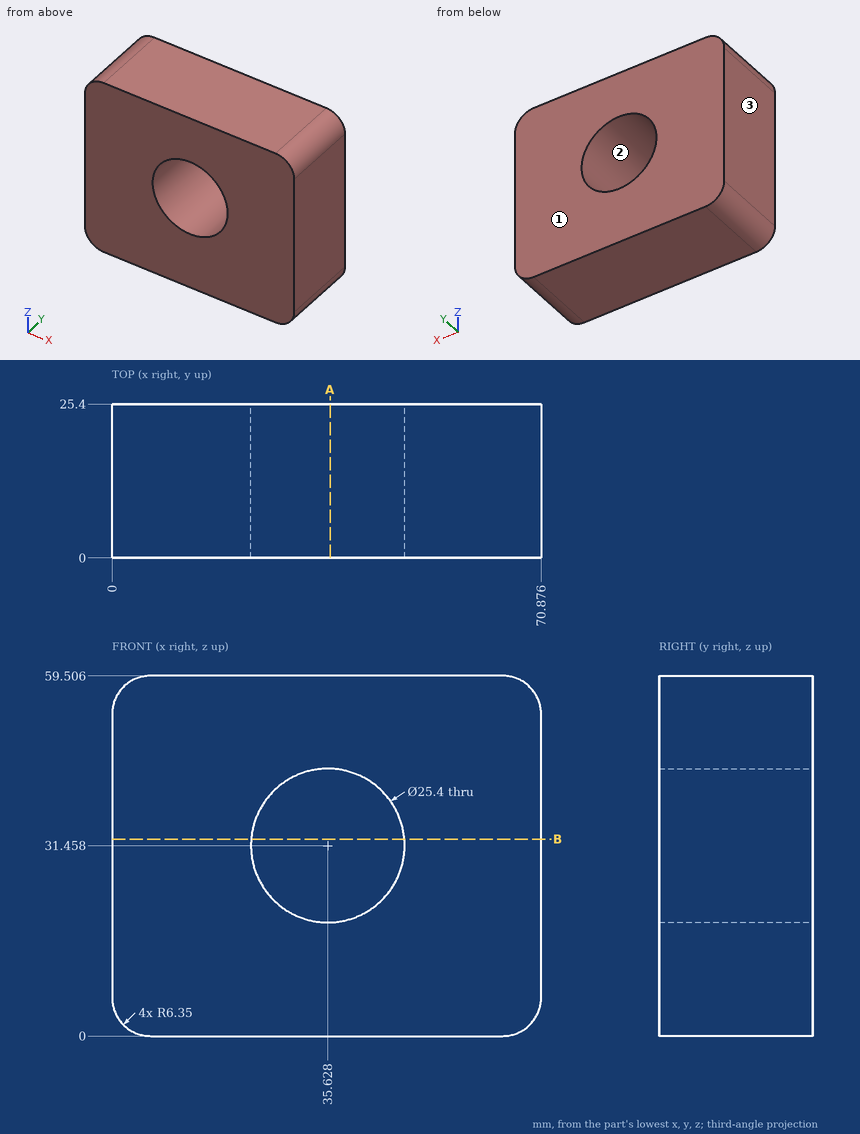
Print and shaded views of the part. All mm, measured from the part's lowest x, y and z. Give positions to 0.01 mm unless a question says otherwise; leave off trailing zeros. Loops run counter-clockwise (first coordinate to the right, second up) from the corner with the lowest first, then second, coordinate; pieces in that order, holes last. Notation, with made-up numbers: (1.25, 19) - (44.25, 19) arc R20 ccw to (44.25, 23) - close; hole circle Ø6 at (48, -22.5). An arc over 180 degrees is marked (long way). One line per item, written item: value. Start each with the question number.
1. Slice it at B-B (z = 32.5). List the corners of the cut face in (x, y) (1 decimal), plus the area to 3 significant figures.
2. Pull direction X, two halves, no side cores. Call the marked faces 1, 2 and 3: pulls with the +X half, pulls with the -X half, needs draft (parallel to the pull), parting line crosses it, or undercut.
3. Probe L1, parallel to Z at x = 6, y = 11.5; L2, parallel to X at y = 16.25, z = 40.5 (1 decimal); L3, parallel to X at y = 16.5, z = 43 (1 decimal). List the from-to ranges inside material, lowest first. Write a range as from..to.
4. Slice it at A-A (x = 36). List the corners of the cut face in (y, z) (1 decimal).
Solution:
1. outline: (0, 0) - (23, 0) - (23, 25.4) - (0, 25.4) - close; (48.3, 0) - (70.9, 0) - (70.9, 25.4) - (48.3, 25.4) - close
1. area: 1,160 mm^2
2. face 1: needs draft
2. face 2: undercut
2. face 3: pulls with the -X half
3. L1: z = 0.01..59.5
3. L2: x = 0..26.7, 44.5..70.9
3. L3: x = 0..30.3, 40.9..70.9
4. outline: (0, 0) - (25.4, 0) - (25.4, 18.8) - (0, 18.8) - close; (0, 44.2) - (25.4, 44.2) - (25.4, 59.5) - (0, 59.5) - close
